```python
from build123d import *

# Parameters (mm, degrees)
BOSS_EXTRUDE1_DEPTH = 0.5


with BuildPart() as part:
    # Sketch1 → Boss-Extrude1 (new body, symmetric)
    with BuildSketch(Plane.XY):
        with BuildLine():
            Line((-17.5, 3), (-17.5, -3))
            Line((-17.5, -3), (-10.472135955, -3))
            ThreePointArc((-10.472135955, -3), (-9.247391084, -2.738612788), (-8.236067977, -2))
            ThreePointArc((-8.236067977, -2), (-7.224744871, -1.261387212), (-6, -1))
            Line((-6, -1), (6, -1))
            ThreePointArc((6, -1), (7.224744871, -1.261387212), (8.236067977, -2))
            ThreePointArc((8.236067977, -2), (9.247391084, -2.738612788), (10.472135955, -3))
            Line((10.472135955, -3), (17.5, -3))
            Line((17.5, -3), (17.5, 3))
            Line((17.5, 3), (10.472135955, 3))
            ThreePointArc((10.472135955, 3), (9.247391084, 2.738612788), (8.236067977, 2))
            ThreePointArc((8.236067977, 2), (7.224744871, 1.261387212), (6, 1))
            Line((6, 1), (-6, 1))
            ThreePointArc((-6, 1), (-7.224744871, 1.261387212), (-8.236067977, 2))
            ThreePointArc((-8.236067977, 2), (-9.247391084, 2.738612788), (-10.472135955, 3))
            Line((-10.472135955, 3), (-17.5, 3))
        make_face()
    extrude(amount=BOSS_EXTRUDE1_DEPTH, both=True)


solid = part.part
```
Verification items for the finished model (mm, model axes). A direction names the side the tool comes from. Coordinates: 2 decimals unless noted, no trailing zeros. Write each loop counter-clockwise with the first axis right and the second up, starting at its lowest first coordinate (ties: lowest second). Pieces come first, ordered by that corner, then holes. Notation, with made-up numbers: M 53.5,19 L 104.5,19 A31 cw 104.5,47 Z; hole C -17.75,69 d4. An arc over 180 degrees is marked long. One line per item, written item: value.
Item 1: Mould release check, pull along X, two halves, no side actions. Record for faces 3 (the flat face through (14, -3, 0)), 4 (the flat face through (-17.5, 0, 0)), 5 (the flat face through (0, -1, 0)): pulls with the +X half, pulls with the -X half, needs draft (parallel to the pull), parting line crosses it, or undercut.
Check sheet entries:
face 3: needs draft
face 4: pulls with the -X half
face 5: undercut
Item 2: Section check C-C, the plane x = 5. Record the boundary of the cut face in (y, z).
Check sheet entries:
outline: M -1,-0.5 L 1,-0.5 L 1,0.5 L -1,0.5 Z
Item 3: Access from +Z, -Z, +X, -X, +Y, -Y to the whole of each face (thin tool, end or side, straight path). Record for faces 1 (the flat face through (0, 1, 0)), 2 (the flat face through (0, 0, 0.5)).
Check sheet entries:
face 1: +Z, -Z, +Y
face 2: +Z, +X, -X, +Y, -Y
Item 4: Section check D-D, the plane x = -9.5. Record the boundary of the cut face in (y, z).
Check sheet entries:
outline: M -2.84,-0.5 L 2.84,-0.5 L 2.84,0.5 L -2.84,0.5 Z
Item 5: Scan lines: line 1 along Y through (x, z) = (-6, -0.2); line 2 along X through (y, z) = (-1.75, -0.4); line 3 along X through (y, z) = (2.45, -0.3). Record each from-to range of solid material in increasing order.
Check sheet entries:
line 1: y = -1 to 1
line 2: x = -17.5 to -7.98, 7.98 to 17.5
line 3: x = -17.5 to -8.74, 8.74 to 17.5
Item 6: Gauge pin test, flat end, axial feed: pin 1 Ø0.5 at (x, z) = (-2, 0) entering from +Y. Record the tip position at first contact, or that the pin passes through.
Check sheet entries:
pin 1: stops at y = 1
Item 7: Section check B-B, the plane z = 0.2. Record the boundary of the cut face in (x, y).
Check sheet entries:
outline: M -17.5,-3 L -10.47,-3 A3 ccw -8.24,-2 A3 cw -6,-1 L 6,-1 A3 cw 8.24,-2 A3 ccw 10.47,-3 L 17.5,-3 L 17.5,3 L 10.47,3 A3 ccw 8.24,2 A3 cw 6,1 L -6,1 A3 cw -8.24,2 A3 ccw -10.47,3 L -17.5,3 Z
Item 8: Section check A-A, the plane y = -1.6. Record the boundary of the cut face in (x, z), plus the area to 3 significant figures.
Check sheet entries:
outline: M -17.5,-0.5 L -7.8,-0.5 L -7.8,0.5 L -17.5,0.5 Z; M 7.8,-0.5 L 17.5,-0.5 L 17.5,0.5 L 7.8,0.5 Z
area: 19.4 mm^2
